Check sheet for the modelled part. Datum: model origin and axes. Units: mm. A direction names the side the tool comes from. Round coordinates to 2 decimals unless told otherwise and drop trailing zeros. Write each loop counter-clockwise with the first axis right and the second up, starting at its lowest first coordinate (ties: lowest second). Pieces come first, ordered by that corner, then holes. Notation, with made-up numbers: (73.25, 1.25) - (132.25, 1.25) arc R19 ccw to (132.25, 10.25) - close; hole circle Ø3 at (11, 33). An arc over 180 degrees is marked (long way). Answer as a JSON object with one key per item and string values. Group by question number.
Item 1: Sectioned sample at C-C on x = 0. Record the boundary of the cut face in (y, z).
Item 2: Sectioned sample at A-A on y = 0. Record the boundary of the cut face in (x, z).
Item 3: Sectioned sample at B-B on x = -17. Record the boundary of the cut face in (y, z).
Item 4: Set-up check for faces 1 (the flat face through (13, -8.75, 67)), 2 (the flat face through (-14, -8.75, 67)), 3 (the flat face through (-13, 8.75, 67)): record each of +Z, -Z, +X, -X, +Y, -Y from which the full face is reachable in a straight line by a thin tool's end or side.
Item 5: Thickness scan on line 1 (Y direction, x = 17, z = 68.2); line 2 (X direction, y = -0.25, z = 57); line 3 (Z direction, x = 13, y = 5.25). Record the ranges inside material, lowest first.
Item 6: Gauge pin test, flat ends, axial feed: P1, Ø2.5, axis at x = 19.5, z = 65, coming from the +Y side; P2, Ø4, axis at y = 1, z = 40.5, coming from the +X side; P3, Ø5, axis at x = -17, y = 0, coming from the -Z side. Record the tip position at first contact, or that the pin passes through.
Item 7: Sectioned sample at D-D on z = 53. Record the boundary of the cut face in (x, y), plus the area to 3 significant figures.
```python
from build123d import *

# Parameters (mm, degrees)
F1_R     = 6.75
F2_DEPTH = 15
F3_R     = 9
F4_DEPTH = 30
F5_R     = 1.6
F6_DEPTH = 6
F7_R     = 3


with BuildPart() as f2:
    # F1 (on offset) → F2 (new body)
    with BuildSketch(Plane.XY.offset(40)):
        Circle(F1_R)
    extrude(amount=-F2_DEPTH)

    # F3 (on offset) → F4 (join)
    with BuildSketch(Plane.XY.offset(40)):
        Circle(F3_R)
    extrude(amount=F4_DEPTH)

    # F5 (on face) → F6 (join)
    with BuildSketch(Plane.XY.offset(70)):
        with BuildLine():
            Line((-2.1065374433, 8.75), (-25, 8.75))
            Line((-25, 8.75), (-25, -8.75))
            Line((-25, -8.75), (-2.1065374433, -8.75))
            ThreePointArc((-2.1065374433, -8.75), (-9, 0), (-2.1065374433, 8.75))
        make_face()
        with Locations((-17, 0)):
            Circle(F5_R, mode=Mode.SUBTRACT)
        with BuildLine():
            Line((25, 8.75), (2.1065374433, 8.75))
            ThreePointArc((2.1065374433, 8.75), (7.0696123299, 5.5696123299), (9, 0))
            ThreePointArc((9, 0), (7.0696123299, -5.5696123299), (2.1065374433, -8.75))
            Line((2.1065374433, -8.75), (25, -8.75))
            Line((25, -8.75), (25, 8.75))
        make_face()
        with Locations((17, 0)):
            Circle(F5_R, mode=Mode.SUBTRACT)
        with BuildLine():
            Line((2.1065374433, -8.75), (-2.1065374433, -8.75))
            ThreePointArc((-2.1065374433, -8.75), (0, -9), (2.1065374433, -8.75))
        make_face()
    extrude(amount=-F6_DEPTH)

    # F7
    f7_edges = [f2.edges().sort_by_distance(p)[0] for p in [
        (7.069612, 5.569612, 64),
        (-9, 0, 64),
        (7.069612, -5.569612, 64),
    ]]
    fillet(f7_edges, radius=F7_R)


solid = f2.part
```
Completed:
{
 "1": {"outline": "(-9, 40) - (-6.75, 40) - (-6.75, 25) - (6.75, 25) - (6.75, 40) - (9, 40) - (9, 70) - (-9, 70) - close"},
 "2": {"outline": "(-25, 64) - (-18.6, 64) - (-18.6, 70) - (-25, 70) - close; (-15.4, 64) - (-12, 64) arc R3 cw to (-9, 61) - (-9, 40) - (-6.75, 40) - (-6.75, 25) - (6.75, 25) - (6.75, 40) - (9, 40) - (9, 61) arc R3 cw to (12, 64) - (15.4, 64) - (15.4, 70) - (-15.4, 70) - close; (18.6, 64) - (25, 64) - (25, 70) - (18.6, 70) - close"},
 "3": {"outline": "(-8.75, 64) - (-1.6, 64) - (-1.6, 70) - (-8.75, 70) - close; (1.6, 64) - (8.75, 64) - (8.75, 70) - (1.6, 70) - close"},
 "4": {"face 1": "+Z, -Z, +X, -Y", "face 2": "+Z, -Z, -X, -Y", "face 3": "+Z, -Z, -X, +Y"},
 "5": {"line 1": "-8.75 to -1.6, 1.6 to 8.75", "line 2": "-9 to 9", "line 3": "64 to 70"},
 "6": {"P1": "y = 8.75", "P2": "x = 9", "P3": "z = 64"},
 "7": {"outline": "circle Ø18 at (0, 0)", "area": "254 mm²"}
}
